Solid Edge part; units mm, degrees
sketch "Sketch1" plane through (0, 0, 0) normal (0, -1, 0) x (1, 0, 0)
  line L0 (5, 2.8868) -> (0, 5.7735)
  line L1 (0, 5.7735) -> (-5, 2.8868)
  line L2 (-5, 2.8868) -> (-5, -2.8868)
  line L3 (-5, -2.8868) -> (0, -5.7735)
  line L4 (0, -5.7735) -> (5, -2.8868)
  line L5 (5, -2.8868) -> (5, 2.8868)
extrude "Protrusion1" add sketch "Sketch1" along normal mid plane 6.4
sketch "Sketch2" plane through (0, 0, 0) normal (1, 0, 0) x (0, 1, 0)
  line L0 (-3.2, 4.35) -> (-2.8186, 5.7735)
revolve "RevolvedCutout1" cut sketch "Sketch2" angle 360 about axis through (0, 0, 0) along (0, -1, 0) material side at (0, -3.0576, 5.0747)
mirror "Mirror1" about plane through (0, 0, 0) normal (0, -1, 0) of "RevolvedCutout1"
hole "孔_7" at (0, -3.2, 0) direction (0, 1, 0) diameter 4.917 end up to next start chamfer 0.6 start chamfer angle 60 end chamfer 0.6 end chamfer angle 60
properties part number "N2611-2312" material "铝 1060"
Input: part model. Units: mm. Frame: model coordinates. Coordinates: 2 decimals unless noted, no trailing zeros. Write each loop counter-clockwise with the first axis right and the second up, starting at its lowest first coordinate (ties: lowest second). Pieces come first, ordered by that corner, then holes. Notation, with made-up numbers: M -6,23 L 16,23 A32 cw 16,57 Z; hole C 29.25,-33 d2. An arc over 180 degrees is marked long. Answer as a JSON object with one key per item and string values. Group by question number.
(1) Section A-A on z = 0. Output: boundary loops of the cut face in (x, y), plus the area to 3 significant figures.
(2) Mould query, pull axis X, two halves, no side actions, for faces 1 (the face through (-3, -3.2, -2)), 2 (the face through (0.738, -0.04, -2.345)), 3 (the face through (2.465, 0.042, -4.35)). Classes: pulls with the +X half, pulls with the -X half, needs draft (parallel to the pull), parting line crosses it, or undercut.
(3) Ray query, line 1 along X through (y, z) = (1.35, 0); line 2 along Z through (x, y) = (-1, 2.5); line 3 along Z through (x, y) = (-0.5, 1). Return the intervals inside material, ascending. Write a range as [from, to].
(4) Contact query for flat-ended pins moving along their axis: P1, Ø3, axis at x = 1, z = -1.5, coming from the -Y side; P2, Ø3, axis at x = 3.5, y = -2, coming from the -Z side; P3, Ø2, axis at x = 1, z = 1.5, coming from the -Y side; P4, Ø5, axis at x = 0, z = 0, coming from the +Y side. Output: stop coordinate, or through.
(5) Section B-B on y = -1.75. Output: boundary loops of the cut face in (x, z), plus the area to 3 significant figures.
Result set:
{
 "1": {"outline": "M -5,-3.03 L -4.35,-3.2 L -3.06,-3.2 L -2.46,-2.85 L -2.46,2.85 L -3.06,3.2 L -4.35,3.2 L -5,3.03 Z; M 2.46,-2.85 L 3.06,-3.2 L 4.35,-3.2 L 5,-3.03 L 5,3.03 L 4.35,3.2 L 3.06,3.2 L 2.46,2.85 Z", "area": "31.9 mm2"},
 "2": {"face 1": "needs draft", "face 2": "undercut", "face 3": "pulls with the +X half"},
 "3": {"line 1": "x = [-5, -2.46], [2.46, 5]", "line 2": "z = [-5.2, -2.25], [2.25, 5.2]", "line 3": "z = [-5.48, -2.41], [2.41, 5.48]"},
 "4": {"P1": "stops at y = -3.2", "P2": "stops at z = -4.62", "P3": "stops at y = -3.05", "P4": "stops at y = 2.88"},
 "5": {"outline": "M -5,-2.89 L 0,-5.77 L 5,-2.89 L 5,2.89 L 0,5.77 L -5,2.89 Z; hole C 0,0 d4.92", "area": "67.6 mm2"}
}
